Study the drawing (mm; zero at the part's minimum x, y, z) and answer. A direction names the side the tool comes from. Round coordinates to 2 decimals unless told otherwise and drop trailing zeros. Order: outer loops, then holes, each group sorted by start corner. A loop starts at its lowest first (then second) coordinate and runs counter-clockwise, first axis right, second up. Notation, with made-up numbers: M 81,-9 L 127,-9 A32 cw 127,17 Z; hole C 77.25,25 d10. An arc over 180 degrees is marked long. Put each result on its own line as item: value. Start each with the question number.
1. The part is cut by section A-A (x = 4). Give the vertices of the cut face in (y, z), then the cut area to 3 significant figures.
2. The part is cut by section B-B (z = 20). Give the vertices of the cut face in (x, y), then the cut area to 3 significant figures.
3. Each of these flat-tipped pins is pushed along its axis until it touches: pin 1 Ø3.5 at (x, z) = (9.34, 14.34) entering from +Y; pin 2 Ø2 at (x, z) = (9.34, 25.66) entering from +Y. Where does it stop, or does it pass through?
4. Consider line 1 (X direction, y = 0.65, z = 20); line 2 (Z direction, x = 16.75, y = 6.25); line 3 (X direction, y = 1.65, z = 28). Determine where each line is inside the solid, lowest interval first.
5. The part is cut by section D-D (x = 23). Give the vertices of the cut face in (y, z).
6. Which of the six approach directions +Z, -Z, +X, -X, +Y, -Y give full straight-line access (tool end or side, diameter ignored) to the marked faces 4 and 5?
7. The part is cut by section C-C (y = 27.2). Give the vertices of the cut face in (x, z), then the cut area to 3 significant figures.
8. The mould has two halves that part along Z. Classify the marked faces 1, 2 and 3: +Z half, -Z half, draft (parallel to the pull), parting line (faces both ways), or undercut.
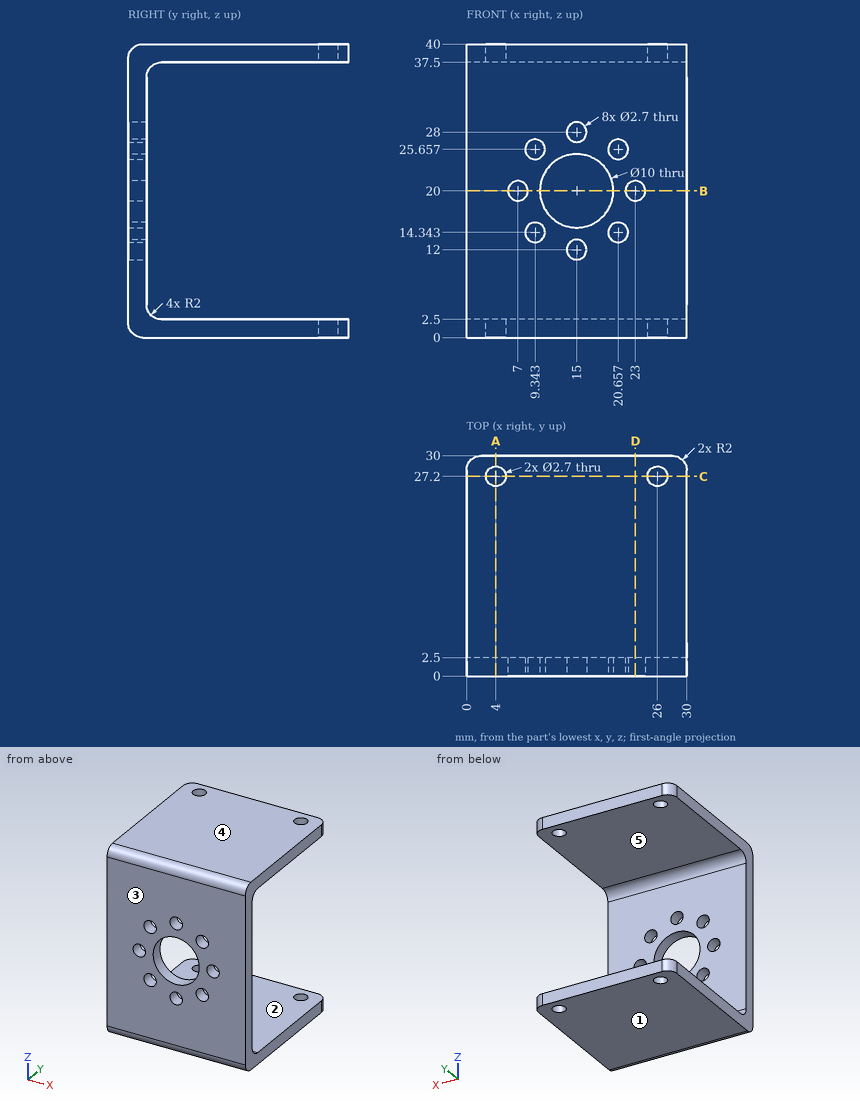
Resolved:
1. outline: M 0,2 A2 ccw 2,0 L 25.85,0 L 25.85,2.5 L 4.5,2.5 A2 cw 2.5,4.5 L 2.5,35.5 A2 cw 4.5,37.5 L 25.85,37.5 L 25.85,40 L 2,40 A2 ccw 0,38 Z; M 28.55,0 L 30,0 L 30,2.5 L 28.55,2.5 Z; M 28.55,37.5 L 30,37.5 L 30,40 L 28.55,40 Z
1. area: 224 mm2
2. outline: M 0,0 L 5.65,0 L 5.65,2.5 L 0,2.5 Z; M 8.35,0 L 10,0 L 10,2.5 L 8.35,2.5 Z; M 20,0 L 21.65,0 L 21.65,2.5 L 20,2.5 Z; M 24.35,0 L 30,0 L 30,2.5 L 24.35,2.5 Z
2. area: 36.5 mm2
3. pin 1: y = 2.5
3. pin 2: through
4. line 1: 0 to 5.65, 8.35 to 10, 20 to 21.65, 24.35 to 30
4. line 2: 0 to 2.5, 37.5 to 40
4. line 3: 0 to 13.65, 16.35 to 30
5. outline: M 0,2 A2 ccw 2,0 L 30,0 L 30,2.5 L 4.5,2.5 A2 cw 2.5,4.5 L 2.5,18.65 L 0,18.65 Z; M 0,21.35 L 2.5,21.35 L 2.5,35.5 A2 cw 4.5,37.5 L 30,37.5 L 30,40 L 2,40 A2 ccw 0,38 Z
6. face 4: +Z, +X, -X, +Y, -Y
6. face 5: +X, -X, +Y
7. outline: M 0,0 L 2.65,0 L 2.65,2.5 L 0,2.5 Z; M 0,37.5 L 2.65,37.5 L 2.65,40 L 0,40 Z; M 5.35,0 L 24.65,0 L 24.65,2.5 L 5.35,2.5 Z; M 5.35,37.5 L 24.65,37.5 L 24.65,40 L 5.35,40 Z; M 27.35,0 L 30,0 L 30,2.5 L 27.35,2.5 Z; M 27.35,37.5 L 30,37.5 L 30,40 L 27.35,40 Z
7. area: 123 mm2
8. face 1: -Z half
8. face 2: undercut
8. face 3: draft
